Geometry check sheet. Reference: the model listing, model coordinates, mm. A direction names the side the tool comes from. Round coordinates to 2 decimals unless told otherwise and drop trailing zeros. Loops run counter-clockwise (first coordinate to the right, second up) from the corner with the lowest first, then second, coordinate; pieces in that order, holes last. Notation, with made-up numbers: (62.5, -22) - (88.5, -22) arc R17 cw to (88.5, 6) - close; hole circle Ø1 at (15, 6.25). An arc over 180 degrees is marked (long way). Answer as CSV lines item,"result". Start each with the question number.
1) Cross-section at A-A on x = -12.4. Record the boundary of the cut face in (y, z), and give its area (3 significant figures).
2) Depth check by flat-ended pin: P1, Ø1.8, axis at x = 28.5, y = 166.5, coming from the -Z side; P2, Ø1.5, axis at y = 124.5, z = 2, coming from the -X side; P3, Ø1.5, axis at x = -34, z = 2, coming from the -Y side. Enter the tip coordinate at first touch or a pass-through.
3) Cross-section at C-C on y = 30. Record the boundary of the cut face in (x, z), and give its area (3 significant figures).
4) Draft check along Y on faces 1 (the cylindrical face through (-22.24, 11.6, 1.52)), 2 (the cylindrical face through (37.93, 51.5, 1.48)), 3 (the cylindrical face through (-12.136, -40.747, 1.521)). Enter one of: released by +Y, released by -Y, zero draft, split by the parting line, or undercut.
5) Thickness scan on line 1 along Y through (x, z) = (-32.4, 1.05); line 2 along Y through (x, z) = (8, 0.7); line 3 along Y through (x, z) = (-29.5, 1.05). Record the ranges inside material, lowest first.
6) Access from +Z, -Z, +X, -X, +Y, -Y to the whole of each face (thin tool, end or side, straight path). Record for faces 4 (the cylindrical face through (17.17, 39.41, 1.48)), 5 (the flat face through (5, 43, 0)).
7) Cross-section at B-B on y = -6.5. Record the boundary of the cut face in (x, z).
8) Cross-section at D-D on z = 2.2. State how many separate pieces and enclosed holes the cut face has, and give its area (3 significant figures).
from build123d import *

# Parameters (mm, degrees)
SKETCH1_W           = 200
SKETCH1_H           = 300
SKETCH1_W_2         = 158.527362204
SKETCH1_H_2         = 20
BOSS_EXTRUDE1_DEPTH = 3
SKETCH2_R           = 2.5
CUT_EXTRUDE1_DEPTH  = 5
CUT_EXTRUDE3_DEPTH  = 10
CUT_EXTRUDE4_REACH  = 183.673
SKETCH5_W           = 62
SKETCH5_H           = 13
FILLET2_R           = 5
FILLET3_R           = 10
FILLET4_R           = 5
CUT_EXTRUDE6_REACH  = 183.673
SKETCH7_R           = 1.6
CUT_EXTRUDE7_REACH  = 183.673
SKETCH8_R           = 2.5
SKETCH8_W           = 20
SKETCH8_H           = 5
FILLET6_R           = 1
FILLET7_R           = 0.5
SKETCH9_R           = 1.5
CUT_EXTRUDE8_DEPTH  = 10
FILLET8_R           = 5


with BuildPart() as part:
    # Sketch1 → Boss-Extrude1 (new body)
    with BuildSketch(Plane.XY):
        Rectangle(SKETCH1_W, SKETCH1_H)
        with Locations((20.736318898, 160)):
            Rectangle(SKETCH1_W_2, SKETCH1_H_2)
    extrude(amount=BOSS_EXTRUDE1_DEPTH)

    # Sketch2 → Cut-Extrude1 (cut)
    with BuildSketch(Plane.XY.offset(3)):
        with Locations((-12.4, -28.75)):
            Circle(SKETCH2_R)
        with Locations((7.6, 11.65)):
            Circle(SKETCH2_R)
        with Locations((-32.4, 11.65)):
            Circle(SKETCH2_R)
        Polygon((-44.5, -3.25), (-44.5, -1.25), (-37.5, -1.25), (-37.5, -13.25), (-39.5, -13.25), (-39.5, -3.25), align=None)
        Polygon((51.5, -3.25), (56.5, -3.25), (56.5, -1.25), (49.5, -1.25), (49.5, -13.25), (51.5, -13.25), align=None)
        with BuildLine():
            Line((-44.5, -3.25), (-44.5, -1.25))
            ThreePointArc((-44.5, -1.25), (-45.5, -2.25), (-44.5, -3.25))
        make_face()
        with BuildLine():
            ThreePointArc((-37.5, -13.25), (-38.5, -14.25), (-39.5, -13.25))
            Line((-39.5, -13.25), (-37.5, -13.25))
        make_face()
        with BuildLine():
            ThreePointArc((51.5, -13.25), (50.5, -14.25), (49.5, -13.25))
            Line((49.5, -13.25), (51.5, -13.25))
        make_face()
        with BuildLine():
            ThreePointArc((56.5, -1.25), (57.5, -2.25), (56.5, -3.25))
            Line((56.5, -3.25), (56.5, -1.25))
        make_face()
    extrude(amount=-CUT_EXTRUDE1_DEPTH, mode=Mode.SUBTRACT)

    # Sketch4 → Cut-Extrude3 (cut)
    with BuildSketch(Plane.XY.offset(3)):
        with BuildLine():
            ThreePointArc((-44.5, -3.25), (-45.5, -2.25), (-44.5, -1.25))
            Line((-44.5, -1.25), (-44.5, 10))
            Line((-44.5, 10), (-52, 10))
            Line((-52, 10), (-52, 50))
            Line((-52, 50), (2.5, 50))
            Line((2.5, 50), (2.5, 170))
            Line((2.5, 170), (-58.527362204, 170))
            Line((-58.527362204, 170), (-58.527362204, 150))
            Line((-58.527362204, 150), (-100, 150))
            Line((-100, 150), (-100, -150))
            Line((-100, -150), (100, -150))
            Line((100, -150), (100, 170))
            Line((100, 170), (36.5, 170))
            Line((36.5, 170), (36.5, 50))
            Line((36.5, 50), (64, 50))
            Line((64, 50), (64, 10))
            Line((64, 10), (56.5, 10))
            Line((56.5, 10), (56.5, -1.25))
            ThreePointArc((56.5, -1.25), (57.5, -2.25), (56.5, -3.25))
            Line((56.5, -3.25), (56.5, -20))
            Line((56.5, -20), (-0.4, -20))
            Line((-0.4, -20), (-0.4, -28.75))
            ThreePointArc((-0.4, -28.75), (-12.4, -40.75), (-24.4, -28.75))
            Line((-24.4, -28.75), (-24.4, -20))
            Line((-24.4, -20), (-44.5, -20))
            Line((-44.5, -20), (-44.5, -3.25))
        make_face()
    extrude(amount=-CUT_EXTRUDE3_DEPTH, mode=Mode.SUBTRACT)

    # Sketch5 → Cut-Extrude4 (cut, up to next)
    with BuildSketch(Plane.XY.offset(3), mode=Mode.PRIVATE) as cut_extrude4_sk1:
        with Locations((-12.4, 34.409289568)):
            Rectangle(SKETCH5_W, SKETCH5_H)
    cut_extrude4_tool1 = extrude(cut_extrude4_sk1.sketch, amount=-CUT_EXTRUDE4_REACH, mode=Mode.PRIVATE) & part.part
    add(cut_extrude4_tool1.solids().sort_by_distance((-12.4, 34.40929, 3))[0], mode=Mode.SUBTRACT)

    # Fillet2
    fillet2_edges = [part.edges().sort_by_distance(p)[0] for p in [
        (-43.4, 40.909289568, 1.5),
        (18.6, 40.909289568, 1.5),
        (18.6, 27.909289568, 1.5),
        (-43.4, 27.909289568, 1.5),
    ]]
    fillet(fillet2_edges, radius=FILLET2_R)

    # Fillet3
    fillet3_edges = [part.edges().sort_by_distance(p)[0] for p in [
        (-52, 50, 1.5),
    ]]
    fillet(fillet3_edges, radius=FILLET3_R)

    # Fillet4
    fillet4_edges = [part.edges().sort_by_distance(p)[0] for p in [
        (-44.5, -20, 1.5),
        (-24.4, -20, 1.5),
        (-0.4, -20, 1.5),
        (56.5, 10, 1.5),
        (64, 50, 1.5),
        (2.5, 50, 1.5),
        (36.5, 50, 1.5),
        (56.5, -20, 1.5),
        (-44.5, 10, 1.5),
    ]]
    fillet(fillet4_edges, radius=FILLET4_R)

    # Sketch7 → Cut-Extrude6 (cut, up to next)
    with BuildSketch(Plane.XY.offset(3), mode=Mode.PRIVATE) as cut_extrude6_sk1:
        with Locations((55.5, 41.3)):
            Circle(SKETCH7_R)
    cut_extrude6_tool1 = extrude(cut_extrude6_sk1.sketch, amount=-CUT_EXTRUDE6_REACH, mode=Mode.PRIVATE) & part.part
    # Sketch7 → Cut-Extrude6 (cut, up to next)
    with BuildSketch(Plane.XY.offset(3), mode=Mode.PRIVATE) as cut_extrude6_sk2:
        with Locations((23.5, 41.3)):
            Circle(SKETCH7_R)
    cut_extrude6_tool2 = extrude(cut_extrude6_sk2.sketch, amount=-CUT_EXTRUDE6_REACH, mode=Mode.PRIVATE) & part.part
    add(cut_extrude6_tool1.solids().sort_by_distance((55.5, 41.3, 3))[0], mode=Mode.SUBTRACT)
    add(cut_extrude6_tool2.solids().sort_by_distance((23.5, 41.3, 3))[0], mode=Mode.SUBTRACT)

    # Sketch8 → Cut-Extrude7 (cut, up to next)
    with BuildSketch(Plane.XY.offset(3), mode=Mode.PRIVATE) as cut_extrude7_sk1:
        with Locations((-4.4, 9.909289568)):
            Circle(SKETCH8_R)
    cut_extrude7_tool1 = extrude(cut_extrude7_sk1.sketch, amount=-CUT_EXTRUDE7_REACH, mode=Mode.PRIVATE) & part.part
    # Sketch8 → Cut-Extrude7 (cut, up to next)
    with BuildSketch(Plane.XY.offset(3), mode=Mode.PRIVATE) as cut_extrude7_sk2:
        with Locations((-20.4, 9.909289568)):
            Circle(SKETCH8_R)
    cut_extrude7_tool2 = extrude(cut_extrude7_sk2.sketch, amount=-CUT_EXTRUDE7_REACH, mode=Mode.PRIVATE) & part.part
    # Sketch8 → Cut-Extrude7 (cut, up to next)
    with BuildSketch(Plane.XY.offset(3), mode=Mode.PRIVATE) as cut_extrude7_sk3:
        with Locations((-12.4, 21.909289568)):
            Rectangle(SKETCH8_W, SKETCH8_H)
    cut_extrude7_tool3 = extrude(cut_extrude7_sk3.sketch, amount=-CUT_EXTRUDE7_REACH, mode=Mode.PRIVATE) & part.part
    add(cut_extrude7_tool1.solids().sort_by_distance((-4.4, 9.90929, 3))[0], mode=Mode.SUBTRACT)
    add(cut_extrude7_tool2.solids().sort_by_distance((-20.4, 9.90929, 3))[0], mode=Mode.SUBTRACT)
    add(cut_extrude7_tool3.solids().sort_by_distance((-12.4, 21.90929, 3))[0], mode=Mode.SUBTRACT)

    # Fillet6
    fillet6_edges = [part.edges().sort_by_distance(p)[0] for p in [
        (-37.5, -1.25, 1.5),
        (49.5, -1.25, 1.5),
    ]]
    fillet(fillet6_edges, radius=FILLET6_R)

    # Fillet7
    fillet7_edges = [part.edges().sort_by_distance(p)[0] for p in [
        (-39.5, -3.25, 1.5),
        (51.5, -3.25, 1.5),
    ]]
    fillet(fillet7_edges, radius=FILLET7_R)

    # Sketch9 → Cut-Extrude8 (cut)
    with BuildSketch(Plane.XY.offset(3)):
        with Locations((10.5, 166.5)):
            Circle(SKETCH9_R)
        with Locations((10.5, 66.5)):
            Circle(SKETCH9_R)
        with Locations((28.5, 166.5)):
            Circle(SKETCH9_R)
        with Locations((28.5, 66.5)):
            Circle(SKETCH9_R)
    extrude(amount=-CUT_EXTRUDE8_DEPTH, mode=Mode.SUBTRACT)

    # Fillet8
    fillet8_edges = [part.edges().sort_by_distance(p)[0] for p in [
        (2.5, 170, 1.5),
        (36.5, 170, 1.5),
        (-52, 10, 1.5),
        (64, 10, 1.5),
    ]]
    fillet(fillet8_edges, radius=FILLET8_R)


solid = part.part
Answer block:
1,outline,"(-40.75, 0) - (-31.25, 0) - (-31.25, 3) - (-40.75, 3) - close; (-26.25, 0) - (19.41, 0) - (19.41, 3) - (-26.25, 3) - close; (24.41, 0) - (27.91, 0) - (27.91, 3) - (24.41, 3) - close; (40.91, 0) - (50, 0) - (50, 3) - (40.91, 3) - close"
1,area,"203 mm^2"
2,P1,"passes through"
2,P2,"stops at x = 2.5"
2,P3,"stops at y = -20"
3,outline,"(-52, 0) - (-42.47, 0) - (-42.47, 3) - (-52, 3) - close; (17.67, 0) - (64, 0) - (64, 3) - (17.67, 3) - close"
3,area,"168 mm^2"
4,face 1,"undercut"
4,face 2,"released by +Y"
4,face 3,"released by -Y"
5,line 1,"y = -20 to 9.15, 14.15 to 27.91, 40.91 to 50"
5,line 2,"y = -20 to 9.18, 14.12 to 27.91, 40.91 to 170"
5,line 3,"y = -20 to 27.91, 40.91 to 50"
6,face 4,"+Z, -Z"
6,face 5,"-Z, +X, -X, +Y, -Y"
7,outline,"(-44.5, 0) - (-39.5, 0) - (-39.5, 3) - (-44.5, 3) - close; (-37.5, 0) - (49.5, 0) - (49.5, 3) - (-37.5, 3) - close; (51.5, 0) - (56.5, 0) - (56.5, 3) - (51.5, 3) - close"
8,separate pieces,"1"
8,enclosed holes,"13"
8,area,"11,100 mm^2"
